from build123d import *

# Parameters (mm, degrees)
SKETCH1_W           = 75
SKETCH1_H           = 95
BOSS_EXTRUDE1_DEPTH = 15
SKETCH2_W           = 95
SKETCH2_H           = 5
BOSS_EXTRUDE2_DEPTH = 5
SKETCH3_R           = 0.6
CUT_EXTRUDE1_DEPTH  = 100
SKETCH4_W           = 5
SKETCH4_H           = 90
CUT_EXTRUDE2_DEPTH  = 100
SKETCH5_W           = 34
SKETCH5_H           = 15
CUT_EXTRUDE3_DEPTH  = 22
SKETCH6_W           = 34
SKETCH6_H           = 15
CUT_EXTRUDE4_DEPTH  = 22
SKETCH7_W           = 37
SKETCH7_H           = 90
CUT_EXTRUDE5_DEPTH  = 13
SKETCH10_W          = 34
SKETCH10_H          = 51
BOSS_EXTRUDE3_DEPTH = 10
SKETCH11_W          = 12.5
SKETCH11_H          = 16.5
CUT_EXTRUDE6_DEPTH  = 100
SKETCH12_W          = 15.5
SKETCH12_H          = 10
CUT_EXTRUDE8_DEPTH  = 100
SKETCH13_W          = 15.75
SKETCH13_H          = 10
CUT_EXTRUDE9_DEPTH  = 7
SKETCH14_W          = 15.75
SKETCH14_H          = 10
CUT_EXTRUDE10_DEPTH = 7
SKETCH15_R          = 1.2
CUT_EXTRUDE11_DEPTH = 100
SKETCH16_R          = 1.2
SKETCH16_W          = 5
SKETCH16_H          = 10
CUT_EXTRUDE12_DEPTH = 100
SKETCH17_R          = 1.5
CUT_EXTRUDE14_DEPTH = 10
FILLET3_R           = 3
FILLET4_R           = 3
SKETCH19_R          = 0.6
CUT_EXTRUDE15_DEPTH = 10


with BuildPart() as part:
    # Sketch1 → Boss-Extrude1 (new body)
    with BuildSketch(Plane(origin=(0, 0, 0), x_dir=(1, 0, 0), z_dir=(0, 1, 0))):
        Rectangle(SKETCH1_W, SKETCH1_H)
    extrude(amount=BOSS_EXTRUDE1_DEPTH)

    # Sketch2 → Boss-Extrude2 (add)
    with BuildSketch(Plane(origin=(37.5, 0, 0), x_dir=(0, 0, -1), z_dir=(1, 0, 0))):
        with Locations((0, 12.5)):
            Rectangle(SKETCH2_W, SKETCH2_H)
    extrude(amount=BOSS_EXTRUDE2_DEPTH)

    # Sketch3 → Cut-Extrude1 (cut)
    with BuildSketch(Plane(origin=(0, 0, -47.5), x_dir=(-1, 0, 0), z_dir=(0, 0, -1))):
        with Locations((-40, 12.458610353)):
            Circle(SKETCH3_R)
    extrude(amount=-CUT_EXTRUDE1_DEPTH, mode=Mode.SUBTRACT)

    # Sketch4 → Cut-Extrude2 (cut)
    with BuildSketch(Plane(origin=(0, 15, 0), x_dir=(1, 0, 0), z_dir=(0, 1, 0))):
        with Locations((40, 0)):
            Rectangle(SKETCH4_W, SKETCH4_H)
    extrude(amount=-CUT_EXTRUDE2_DEPTH, mode=Mode.SUBTRACT)

    # Sketch5 → Cut-Extrude3 (cut)
    with BuildSketch(Plane(origin=(0, 0, -47.5), x_dir=(-1, 0, 0), z_dir=(0, 0, -1))):
        with Locations((20.5, 7.5)):
            Rectangle(SKETCH5_W, SKETCH5_H)
    extrude(amount=-CUT_EXTRUDE3_DEPTH, mode=Mode.SUBTRACT)

    # Sketch6 → Cut-Extrude4 (cut)
    with BuildSketch(Plane.XY.offset(47.5)):
        with Locations((-20.5, 7.5)):
            Rectangle(SKETCH6_W, SKETCH6_H)
    extrude(amount=-CUT_EXTRUDE4_DEPTH, mode=Mode.SUBTRACT)

    # Sketch7 → Cut-Extrude5 (cut)
    with BuildSketch(Plane(origin=(0, 15, 0), x_dir=(1, 0, 0), z_dir=(0, 1, 0))):
        with Locations((17, 0)):
            Rectangle(SKETCH7_W, SKETCH7_H)
    extrude(amount=-CUT_EXTRUDE5_DEPTH, mode=Mode.SUBTRACT)

    # Sketch10 → Boss-Extrude3 (add)
    with BuildSketch(Plane(origin=(0, 15, 0), x_dir=(1, 0, 0), z_dir=(0, 1, 0))):
        with Locations((-20.5, 0)):
            Rectangle(SKETCH10_W, SKETCH10_H)
    extrude(amount=BOSS_EXTRUDE3_DEPTH)

    # Sketch11 → Cut-Extrude6 (cut)
    with BuildSketch(Plane.XY.offset(25.5)):
        with Locations((-19.5, 10.25)):
            Rectangle(SKETCH11_W, SKETCH11_H)
    extrude(amount=-CUT_EXTRUDE6_DEPTH, mode=Mode.SUBTRACT)

    # Sketch12 → Cut-Extrude8 (cut)
    with BuildSketch(Plane.ZY.offset(37.5)):
        with Locations((0, 20)):
            Rectangle(SKETCH12_W, SKETCH12_H)
    extrude(amount=-CUT_EXTRUDE8_DEPTH, mode=Mode.SUBTRACT)

    # Sketch13 → Cut-Extrude9 (cut)
    with BuildSketch(Plane.ZY.offset(37.5)):
        with Locations((-17.625, 20)):
            Rectangle(SKETCH13_W, SKETCH13_H)
    extrude(amount=-CUT_EXTRUDE9_DEPTH, mode=Mode.SUBTRACT)

    # Sketch14 → Cut-Extrude10 (cut)
    with BuildSketch(Plane.ZY.offset(37.5)):
        with Locations((17.625, 20)):
            Rectangle(SKETCH14_W, SKETCH14_H)
    extrude(amount=-CUT_EXTRUDE10_DEPTH, mode=Mode.SUBTRACT)

    # Sketch15 → Cut-Extrude11 (cut)
    with BuildSketch(Plane.XY.offset(9.75)):
        with Locations((-34, 20)):
            Circle(SKETCH15_R)
    extrude(amount=-CUT_EXTRUDE11_DEPTH, mode=Mode.SUBTRACT)

    # Sketch16 → Cut-Extrude12 (cut)
    with BuildSketch(Plane(origin=(0, 2, 0), x_dir=(1, 0, 0), z_dir=(0, 1, 0))):
        with Locations(Location((31, 30, 0), (0, 0, 270))):
            Circle(SKETCH16_R)
        with Locations(Location((31, -30, 0), (0, 0, 270))):
            Circle(SKETCH16_R)
        with Locations((31, -38)):
            Rectangle(SKETCH16_W, SKETCH16_H)
        with Locations((31, 38)):
            Rectangle(SKETCH16_W, SKETCH16_H)
    extrude(amount=-CUT_EXTRUDE12_DEPTH, mode=Mode.SUBTRACT)

    # Sketch17 → Cut-Extrude14 (cut)
    with BuildSketch(Plane(origin=(0, 25, 0), x_dir=(1, 0, 0), z_dir=(0, 1, 0))):
        with Locations(Location((-20, -16.625, 0), (0, 0, 270))):
            Circle(SKETCH17_R)
        with Locations(Location((-20, 16.625, 0), (0, 0, 270))):
            Circle(SKETCH17_R)
    extrude(amount=-CUT_EXTRUDE14_DEPTH, mode=Mode.SUBTRACT)

    # Fillet3
    # the kernel refuses this fillet: 3 mm, written as the material it adds along each edge
    with BuildSketch(Plane(origin=(-3.5, 15, -25.5), x_dir=(1, 0, 0), z_dir=(0, 0, 1))) as fillet3_piece_1:
        with BuildLine():
            CenterArc((3, 2.828427125), FILLET3_R, 180, 70.528779366)
            Line((0, 2.828427125), (0, 0))
            Line((0, 0), (2, 0))
        make_face()
    extrude(amount=17.75)
    # the kernel refuses this fillet: 3 mm, written as the material it takes off along each edge
    with BuildSketch(Plane(origin=(-3.5, 25, -33), x_dir=(-1, 0, 0), z_dir=(0, 0, 1))) as fillet3_2_piece_1:
        with BuildLine():
            CenterArc((FILLET3_R, FILLET3_R), FILLET3_R, 180, 90)
            Line((0, FILLET3_R), (0, 0))
            Line((0, 0), (FILLET3_R, 0))
        make_face()
    extrude(amount=32.75, mode=Mode.SUBTRACT)

    # Fillet4
    # the kernel refuses this fillet: 3 mm, written as the material it adds along each edge
    with BuildSketch(Plane(origin=(-3.5, 15, 7.75), x_dir=(1, 0, 0), z_dir=(0, 0, 1))) as fillet4_piece_1:
        with BuildLine():
            CenterArc((3, 2.828427125), FILLET4_R, 180, 70.528779366)
            Line((0, 2.828427125), (0, 0))
            Line((0, 0), (2, 0))
        make_face()
    extrude(amount=17.75)
    # the kernel refuses this fillet: 3 mm, written as the material it takes off along each edge
    with BuildSketch(Plane(origin=(-3.5, 25, 0.25), x_dir=(-1, 0, 0), z_dir=(0, 0, 1))) as fillet4_2_piece_1:
        with BuildLine():
            CenterArc((FILLET4_R, FILLET4_R), FILLET4_R, 180, 90)
            Line((0, FILLET4_R), (0, 0))
            Line((0, 0), (FILLET4_R, 0))
        make_face()
    extrude(amount=32.75, mode=Mode.SUBTRACT)

    # Sketch19 → Cut-Extrude15 (cut)
    with BuildSketch(Plane(origin=(37.5, 0, 0), x_dir=(0, 0, -1), z_dir=(1, 0, 0))):
        with Locations((0, 8)):
            Circle(SKETCH19_R)
    extrude(amount=-CUT_EXTRUDE15_DEPTH, mode=Mode.SUBTRACT)


solid = part.part
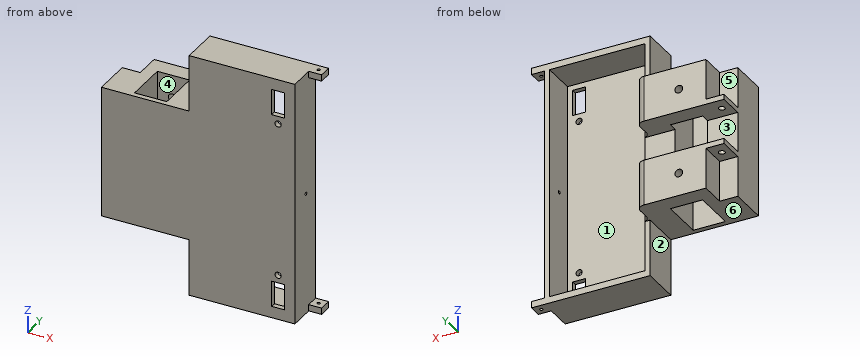
The listing builds one solid part. Answer for the finished solid, in the listing's coordinates (mm). Face numbers are marked on the shaded views. A direction names the side the tool comes from. Give positions to 0.01 mm unless a question says otherwise; leave off trailing zeros. Loops run counter-clockwise (first coordinate to the right, second up) from the corner with the lowest first, then second, coordinate; pieces in that order, holes last.
Item 1: A tool of negligible diameter and unlimited length cuts with its end or side. For the marked faces 1, 2 and 3, from which of +Z, -Z, +X, -X, +Y, -Y can it reach the whole face along a straight path? Write none if from no direction.
Derived:
face 1: +Y
face 2: -Z, -X, +Y, -Y
face 3: +X, -X, +Y
Item 2: A cutting plane is placed at D-D (z = 38). Give the vertices of the cut face in (x, y), then the cut area to 3 significant figures.
Derived:
outline: (-3.5, 0) - (28.5, 0) - (28.5, 2) - (-1.5, 2) - (-1.5, 15) - (-3.5, 15) - close; (33.5, 0) - (37.5, 0) - (37.5, 15) - (35.5, 15) - (35.5, 2) - (33.5, 2) - close
area: 124 mm2
Item 3: Each of these flat-tipped pins is pushed along its axis until it touches: pin 1 Ø4 at (x, y) = (-34, 20) entering from -Z; pin 2 Ø4 at (x, y) = (-7, 9) entering from +Z; pin 3 Ø0.6 at (y, z) = (1, 40) entering from -X. Where does it stop, or does it pass through?
Derived:
pin 1: stops at z = -9.75
pin 2: stops at z = 25.5
pin 3: stops at x = -3.5
Item 4: Find the intervals of material crossed by line 1 along X through (y, z) = (8, 24); line 2 along X through (y, z) = (17.75, -12); line 3 along Z through (x, y) = (-12, 20.75), in increasing order.
Derived:
line 1: x = -37.5 to -25.75, -13.25 to -1.5, 35.5 to 37.5
line 2: x = -30.5 to -25.75, -13.25 to -3.5
line 3: z = -25.5 to -7.75, 7.75 to 25.5
Item 5: A cutting plane is placed at C-C (y = 20). Give the vertices of the cut face in (x, z) (3 decimals).
Derived:
outline: (-37.5, -9.75) - (-35.2, -9.75) - (-35.2, -7.75) - (-37.5, -7.75) - close; (-37.5, 7.75) - (-35.2, 7.75) - (-35.2, 9.75) - (-37.5, 9.75) - close; (-32.8, -9.75) - (-30.5, -9.75) - (-30.5, -25.5) - (-3.5, -25.5) - (-3.5, -7.75) - (-32.8, -7.75) - close; (-32.8, 7.75) - (-3.5, 7.75) - (-3.5, 25.5) - (-30.5, 25.5) - (-30.5, 9.75) - (-32.8, 9.75) - close; hole circle Ø3 at (-20, -16.625); hole circle Ø3 at (-20, 16.625)
Item 6: A cutting plane is placed at A-A (y = 5). Give the vertices of the cut face in (x, z).
Derived:
outline: (-37.5, -25.5) - (-25.75, -25.5) - (-25.75, 25.5) - (-37.5, 25.5) - close; (-13.25, -25.5) - (-3.5, -25.5) - (-3.5, -47.5) - (37.5, -47.5) - (37.5, 47.5) - (-3.5, 47.5) - (-3.5, 25.5) - (-13.25, 25.5) - close; hole (-1.5, -45) - (35.5, -45) - (35.5, 45) - (-1.5, 45) - close
Item 7: A cutting plane is placed at B-B (x = -20). Give the vertices of the cut face in (y, z) (3 decimals), then the cut area to 3 significant figures.
Derived:
outline: (0, -25.5) - (2, -25.5) - (2, 25.5) - (0, 25.5) - close; (18.5, -25.5) - (25, -25.5) - (25, -18.125) - (18.5, -18.125) - close; (18.5, -15.125) - (25, -15.125) - (25, -7.75) - (18.5, -7.75) - close; (18.5, 7.75) - (25, 7.75) - (25, 15.125) - (18.5, 15.125) - close; (18.5, 18.125) - (25, 18.125) - (25, 25.5) - (18.5, 25.5) - close
area: 294 mm2
Item 8: Determine the mould class of the marked faces 4, 5 and 6 for opening direction Y: +Y half, -Y half, draft (parallel to the pull), parting line (faces both ways), or undercut.
Derived:
face 4: undercut
face 5: +Y half
face 6: draft
